Work out the finished part from the listing and answer in its coordinate system (mm). A direction names the side the tool comes from. Round coordinates to 2 decimals unless told otherwise and drop trailing zeros. Write each loop counter-clockwise with the first axis right and the second up, starting at its lowest first coordinate (ties: lowest second). Pieces come first, ordered by that corner, then holes.
1. Find section A-A (y = 27.5). Write down the section's boundary in (x, z), and give its area (3 significant figures).
2. Find section C-C (z = -5.5). Write down the section's boundary in (x, y), and give its area (3 significant figures).
3. Determine the mould class of faces 1 (the face through (-6, -0.46, -28.69)), 2 (the face through (10, 0, 0)), 3 (the face through (0, 0, 35)) for opening direction Z: pulls with the +Z half, pulls with the -Z half, needs draft (parallel to the pull), parting line crosses it, or undercut.
4. A tool of negligible diameter and unlimited length cuts with its end or side. For faces 4 (the face through (-9, -32.5, 0)), 5 (the face through (0, 0, -20)), from which of +Z, -Z, +X, -X, +Y, -Y can it reach the whole face along a straight path? Write none if from no direction.
5. Find section B-B (x = 0). Write down the section's boundary in (y, z).
6. Find section D-D (z = 30). Write down the section's boundary in (x, y).
7. Straight lines are drawn through the part: probe 1 along X at (y, z) = (-6, -30); probe 2 along Z at (x, y) = (-0.5, 15); probe 3 along X at (y, z) = (-7, -12). For each, find the intervals that lie inside material, in ascending order.
```python
from build123d import *

# Parameters (mm, degrees)
SKETCH1_W             = 20
SKETCH1_H             = 70
BOSS_EXTRUDE1_DEPTH   = 32.5
CUT_EXTRUDE1_DEPTH    = 75.498322129
SKETCH3_R             = 1.5
CUT_EXTRUDE2_DEPTH    = 100
M4_TAPPED_HOLE1_D     = 3.3
M4_TAPPED_HOLE1_DEPTH = 102.1
M4_TAPPED_HOLE1_TIP   = 0.991420021


with BuildPart() as part:
    # Sketch1 → Boss-Extrude1 (new, symmetric)
    with BuildSketch(Plane(origin=(0, 0, 0), x_dir=(1, 0, 0), z_dir=(0, 1, 0))):
        Rectangle(SKETCH1_W, SKETCH1_H)
    extrude(amount=BOSS_EXTRUDE1_DEPTH, both=True)

    # Sketch2 → Cut-Extrude1 (cut, through all)
    with BuildSketch(Plane.XZ.offset(32.5)):
        with BuildLine():
            Line((-7.5, -12.5), (-7.5, 12.5))
            ThreePointArc((-7.5, 12.5), (0, 20), (7.5, 12.5))
            Line((7.5, 12.5), (7.5, -12.5))
            ThreePointArc((7.5, -12.5), (0, -20), (-7.5, -12.5))
        make_face()
    extrude(amount=-CUT_EXTRUDE1_DEPTH, mode=Mode.SUBTRACT)

    # Sketch3 → Cut-Extrude2 (cut)
    with BuildSketch(Plane.XZ.offset(32.5)):
        with Locations(Location((5, 30, 0), (0, 0, 270))):
            Circle(SKETCH3_R)
        with Locations(Location((-5, 30, 0), (0, 0, 90))):
            Circle(SKETCH3_R)
        with Locations(Location((5, -30, 0), (0, 0, 90))):
            Circle(SKETCH3_R)
        with Locations(Location((-5, -30, 0), (0, 0, 270))):
            Circle(SKETCH3_R)
    extrude(amount=-CUT_EXTRUDE2_DEPTH, mode=Mode.SUBTRACT)

    # M4 Tapped Hole1
    with Locations(Plane(origin=(-5, 32.5, 30), x_dir=(0, 0, 1), z_dir=(0, 1, 0))):
        with Locations((0, 0), (0, 10), (-60, 10), (-60, 0)):
            Hole(M4_TAPPED_HOLE1_D / 2, depth=M4_TAPPED_HOLE1_DEPTH)
            with Locations((0, 0, -(M4_TAPPED_HOLE1_DEPTH + M4_TAPPED_HOLE1_TIP / 2))):  # 118° drill point
                Cone(0, M4_TAPPED_HOLE1_D / 2, M4_TAPPED_HOLE1_TIP, mode=Mode.SUBTRACT)


solid = part.part
```
Worked answers:
1. outline: (-10, -35) - (10, -35) - (10, 35) - (-10, 35) - close; hole (-7.5, -12.5) arc R7.5 ccw to (7.5, -12.5) - (7.5, 12.5) arc R7.5 ccw to (-7.5, 12.5) - close; hole circle Ø3.3 at (-5, -30); hole circle Ø3.3 at (-5, 30); hole circle Ø3.3 at (5, -30); hole circle Ø3.3 at (5, 30)
1. area: 814 mm2
2. outline: (-10, -32.5) - (-7.5, -32.5) - (-7.5, 32.5) - (-10, 32.5) - close; (7.5, -32.5) - (10, -32.5) - (10, 32.5) - (7.5, 32.5) - close
2. area: 325 mm2
3. face 1: undercut
3. face 2: needs draft
3. face 3: pulls with the +Z half
4. face 4: +Z, -Z, +X, -X, -Y
4. face 5: +Y, -Y
5. outline: (-32.5, -35) - (32.5, -35) - (32.5, -20) - (-32.5, -20) - close; (-32.5, 20) - (32.5, 20) - (32.5, 35) - (-32.5, 35) - close
6. outline: (-10, -32.5) - (-6.65, -32.5) - (-6.65, 32.5) - (-10, 32.5) - close; (-3.35, -32.5) - (3.35, -32.5) - (3.35, 32.5) - (-3.35, 32.5) - close; (6.65, -32.5) - (10, -32.5) - (10, 32.5) - (6.65, 32.5) - close
7. probe 1: x = -10 to -6.65, -3.35 to 3.35, 6.65 to 10
7. probe 2: z = -35 to -19.98, 19.98 to 35
7. probe 3: x = -10 to -7.5, 7.5 to 10
